Here's how the part is built. I have some questions about the finished solid (model axes, mm). Face numbers are marked on the shaded views. A direction names the side the tool comes from. Round coordinates to 2 decimals unless told otherwise and drop trailing zeros. Order: outer loops, then holes, each group sorted by start corner. A loop starts at its lowest first (then second) coordinate and runs counter-clockwise, first axis right, second up. Notation, with made-up numbers: (-20.5, -3.5) -> (-11.5, -3.5) arc R10 cw to (-11.5, 5.5) -> close; hole circle Ø9 at (56.25, -17.5). An arc over 180 degrees is marked (long way). Use a Markdown table: item, result. Add a question column.
(1) On a 3-axis mill with a long thin cutter (end or side, diameter ignored), from which of +Z, -Z, +X, -X, +Y, -Y can I reach the whole of each face in a straight line? I mean the marked faces 4, 5 and 6. Say none if no direction works.
(2) I want a section at B-B, the plane y = -32.5. Please give me the cut outline in (x, z).
(3) Thinking about a two-plate mould opening in Y: for the marked faces 1, 2 and 3, which applies, pulls with the +Y half, pulls with the -Y half, needs draft (parallel to the pull), parting line crosses it, or undercut?
(4) If I drill on probe 1 along Y at (x, z) = (3, 9.5); probe 2 along X at (y, z) = (-43, 0.75); probe 3 along Y at (x, z) = (7, 9.5), over which ranges is the centre line in solid material (lowest first)?
(5) I'm going to push flat-ended pins straight in: P1, Ø0.9, axis at x = 26, z = 4, coming from the -Y side; P2, Ø2.5, axis at x = 15.5, z = 4, coming from the -Y side. Where does each tip first touch, or does it pass through?
(6) I want a section at A-A, the plane z = 4.5. Give the number of separate pieces and of enclosed holes in the cut face, then the cut area to 3 significant figures.
(7) I want a section at D-D, the plane x = 15. Please give me the cut outline in (y, z), then the cut area to 3 significant figures.
(8) I want a section at C-C, the plane x = 6. Please give me the cut outline in (y, z), then the cut area to 3 significant figures.
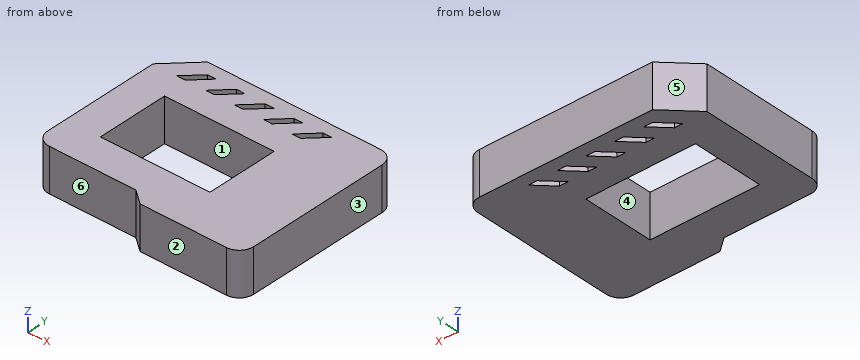
from build123d import *

# Parameters (mm, degrees)
EXTRUDE_1_DEPTH     = 15
FILLET_1_R          = 5
CUT_EXTRUDE_1_DEPTH = 90.724081338
SKETCH_4_W          = 38
SKETCH_4_H          = 25
CUT_EXTRUDE_2_DEPTH = 90.724081338


with BuildPart() as part:
    # 草图1 → 凸台-拉伸1 (new body)
    with BuildSketch(Plane.XY):
        Polygon((-9.999515105, -56.002897725), (25.000484895, -56.002897725), (30.000484895, -60.002897725), (65.000484895, -60.002897725), (65.000484895, -0.002897725), (0.000484895, -0.002897725), (-9.999515105, -10.002897725), align=None)
    extrude(amount=EXTRUDE_1_DEPTH)

    # 圆角1
    fillet_1_edges = [part.edges().sort_by_distance(p)[0] for p in [
        (-9.999515105, -56.002897725, 7.5),
        (65.000484895, -0.002897725, 7.5),
        (65.000484895, -60.002897725, 7.5),
    ]]
    fillet(fillet_1_edges, radius=FILLET_1_R)

    # 草图3 → 切除-拉伸1 (cut, through all)
    with BuildSketch(Plane.XY.offset(15)):
        Polygon((3.856343928, -4.346043475), (-1.800510321, -10.002897725), (1.199489679, -10.002897725), (6.856343928, -4.346043475), align=None)
        Polygon((16.856343928, -4.346043475), (11.199489679, -10.002897725), (8.199489679, -10.002897725), (13.856343928, -4.346043475), align=None)
        Polygon((26.856343928, -4.346043475), (21.199489679, -10.002897725), (18.199489679, -10.002897725), (23.856343928, -4.346043475), align=None)
        Polygon((36.856343928, -4.346043475), (31.199489679, -10.002897725), (28.199489679, -10.002897725), (33.856343928, -4.346043475), align=None)
        Polygon((46.856343928, -4.346043475), (41.199489679, -10.002897725), (38.199489679, -10.002897725), (43.856343928, -4.346043475), align=None)
    extrude(amount=-CUT_EXTRUDE_1_DEPTH, mode=Mode.SUBTRACT)

    # 草图4 → 切除-拉伸2 (cut, through all)
    with BuildSketch(Plane.XY.offset(15)):
        with Locations((21.000484895, -31.502897725)):
            Rectangle(SKETCH_4_W, SKETCH_4_H)
    extrude(amount=-CUT_EXTRUDE_2_DEPTH, mode=Mode.SUBTRACT)


solid = part.part
Taken from the geometry:
| question | item | result |
|---|---|---|
| 1 | face 4 | +Z, -Z |
| 1 | face 5 | +Z, -Z, -X, +Y |
| 1 | face 6 | +Z, -Z, -X, -Y |
| 2 | outline | (-10, 0) -> (2, 0) -> (2, 15) -> (-10, 15) -> close; (40, 0) -> (65, 0) -> (65, 15) -> (40, 15) -> close |
| 3 | face 1 | undercut |
| 3 | face 2 | pulls with the -Y half |
| 3 | face 3 | needs draft |
| 4 | probe 1 | y = -56 to -44, -19 to -8.2, -5.2 to 0 |
| 4 | probe 2 | x = -10 to 2, 40 to 65 |
| 4 | probe 3 | y = -56 to -44, -19 to 0 |
| 5 | P1 | stops at y = -57.16 |
| 5 | P2 | stops at y = -56 |
| 6 | separate pieces | 1 |
| 6 | enclosed holes | 6 |
| 6 | area | 3,250 mm2 |
| 7 | outline | (-56, 0) -> (-44, 0) -> (-44, 15) -> (-56, 15) -> close; (-19, 0) -> (-6.2, 0) -> (-6.2, 15) -> (-19, 15) -> close; (-4.35, 0) -> (0, 0) -> (0, 15) -> (-4.35, 15) -> close |
| 7 | area | 437 mm2 |
| 8 | outline | (-56, 0) -> (-44, 0) -> (-44, 15) -> (-56, 15) -> close; (-19, 0) -> (-5.2, 0) -> (-5.2, 15) -> (-19, 15) -> close; (-4.35, 0) -> (0, 0) -> (0, 15) -> (-4.35, 15) -> close |
| 8 | area | 452 mm2 |
